Geometry check sheet. Reference: drawing and pictorial views, mm from the part's lowest x, y, z. A direction names the side the tool comes from. Round coordinates to 2 decimals unless told otherwise and drop trailing zeros. Loops run counter-clockwise (first coordinate to the right, second up) from the corner with the lowest first, then second, coordinate; pieces in that order, holes last. Notation, with made-up numbers: (80, 39) - (107, 39) arc R18 cw to (107, 61) - close; hole circle Ø10 at (14, 83). An arc over 180 degrees is marked (long way). Put each result on its own line as item: value. Start each with the question number.
Item 1: Draft check along Y on the marked faces 1, 2, 3 and 4. Enter one of: pulls with the +Y half, pulls with the -Y half, needs draft (parallel to the pull), parting line crosses it, or undercut.
Item 2: Gauge pin test, flat ends, axial feed: pin 1 Ø4.5 at (x, y) = (31.75, 3.97) entering from +Z (1 decimal); pin 2 Ø3 at (x, y) = (32.5, 5.5) entering from +Z (1 decimal). Record the tip position at first contact, or that the pin passes through.
Item 3: Section check C-C, the plane z = 4.5. Record the cut outline in (x, y), and give its area (3 significant figures).
Item 4: Tool access check on the marked faces 5 and 6. Record the directions out of +Z, -Z, +X, -X, +Y, -Y that give a thin tool (end or side, any length) a straight path to the whole face; none if there is none.
Item 5: Section check A-A, the plane y = 4.75. Give the number of separate pieces and of enclosed holes in the cut face, and give its area (3 significant figures).
Item 6: Material ranges on line 1 along X through (y, z) = (2.5, 1.5) (1 decimal); line 2 along Y through (x, z) = (6.35, 5.65); line 3 along X through (y, z) = (4.5, 2.5), recorded low to high.
Item 7: Section check B-B, the plane x = 31.75. Record the cut outline in (y, z) (1 decimal).
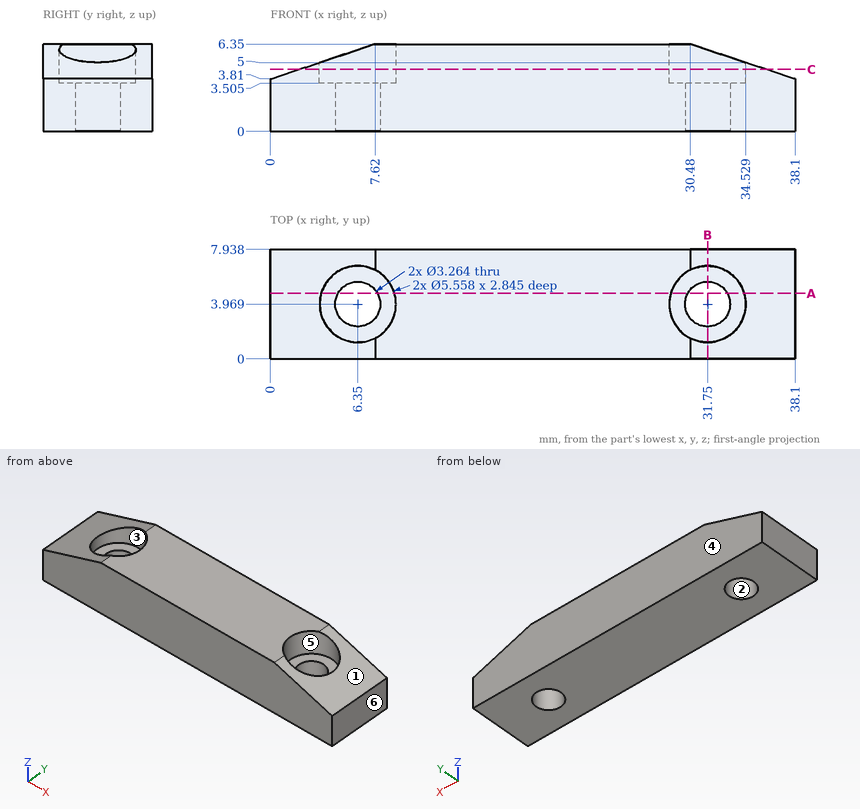
Check result:
1. face 1: needs draft
1. face 2: undercut
1. face 3: undercut
1. face 4: pulls with the +Y half
2. pin 1: z = 3.5
2. pin 2: z = 6
3. outline: (2.07, 0) - (36.03, 0) - (36.03, 7.94) - (2.07, 7.94) - close; hole circle Ø5.56 at (6.35, 3.97); hole circle Ø5.56 at (31.75, 3.97)
3. area: 221 mm²
4. face 5: +Z
4. face 6: +Z, -Z, +X, +Y, -Y
5. separate pieces: 3
5. enclosed holes: 0
5. area: 177 mm²
6. line 1: 0 to 5.6, 7.1 to 31, 32.5 to 38.1
6. line 2: 0 to 1.19, 6.75 to 7.94
6. line 3: 0 to 4.81, 7.89 to 30.21, 33.29 to 38.1
7. outline: (0, 0) - (2.3, 0) - (2.3, 3.5) - (1.2, 3.5) - (1.2, 5.9) - (0, 5.9) - close; (5.6, 0) - (7.9, 0) - (7.9, 5.9) - (6.7, 5.9) - (6.7, 3.5) - (5.6, 3.5) - close
